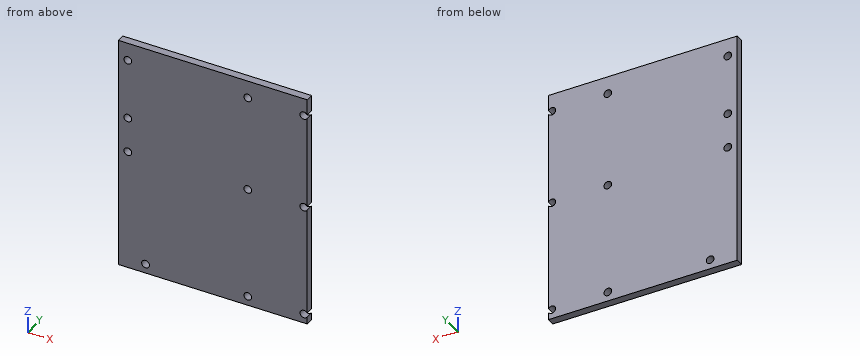
from build123d import *

# Parameters (mm, degrees)
SKETCH2_W           = 243.84
SKETCH2_H           = 304.8
BOSS_EXTRUDE1_DEPTH = 10
SKETCH1_R           = 5
CUT_EXTRUDE2_DEPTH  = 10


with BuildPart() as part:
    # Sketch2 → Boss-Extrude1 (new body)
    with BuildSketch(Plane(origin=(0, 0, 0), x_dir=(1, 0, 0), z_dir=(0, 1, 0))):
        Rectangle(SKETCH2_W, SKETCH2_H)
    extrude(amount=BOSS_EXTRUDE1_DEPTH)

    # Sketch1 → Cut-Extrude2 (cut)
    with BuildSketch(Plane(origin=(0, 0, 0), x_dir=(1, 0, 0), z_dir=(0, 1, 0))):
        with Locations((-86.9, 140.24)):
            Circle(SKETCH1_R)
        with Locations((45.18, 140.24)):
            Circle(SKETCH1_R)
        with Locations((117.57, 140.24)):
            Circle(SKETCH1_R)
        with Locations((117.57, -5.08)):
            Circle(SKETCH1_R)
        with Locations((45.18, -5.08)):
            Circle(SKETCH1_R)
        with Locations((-109.76, -5.08)):
            Circle(SKETCH1_R)
        with Locations((-109.76, -50.8)):
            Circle(SKETCH1_R)
        with Locations((-109.76, -129.196094703)):
            Circle(SKETCH1_R)
        with Locations((45.18, -129.54)):
            Circle(SKETCH1_R)
        with Locations((117.57, -129.54)):
            Circle(SKETCH1_R)
    extrude(amount=CUT_EXTRUDE2_DEPTH, mode=Mode.SUBTRACT)


solid = part.part
The model under review builds one solid part; all positions refer to its coordinate system, in mm. Round coordinates to 2 decimals unless told otherwise and drop trailing zeros. Loops run counter-clockwise (first coordinate to the right, second up) from the corner with the lowest first, then second, coordinate; pieces in that order, holes last. Notation, with made-up numbers: M -11,67 L 17,67 A16 cw 17,85 Z; hole C 9.5,27 d4. An arc over 180 degrees is marked long. Answer as a JSON object with one key per item and string values.
Item 1: For line 1 along Z through (x, y) = (117.57, 4.75); line 2 along X through (y, z) = (2, 5.08); line 3 along Z through (x, y) = (-109.76, 5.5), list the stretches that pass through material, from the lowest coordinate up.
Check sheet entries:
{"line 1": "-152.4 to -145.24, -135.24 to 0.08, 10.08 to 124.54, 134.54 to 152.4", "line 2": "-121.92 to -114.76, -104.76 to 40.18, 50.18 to 112.57", "line 3": "-152.4 to 0.08, 10.08 to 45.8, 55.8 to 124.2, 134.2 to 152.4"}
Item 2: We need section C-C, the plane x = -86.9. State the section outline as (y, z) points, and give its area (3 significant figures).
Check sheet entries:
{"outline": "M 0,-152.4 L 10,-152.4 L 10,-145.24 L 0,-145.24 Z; M 0,-135.24 L 10,-135.24 L 10,152.4 L 0,152.4 Z", "area": "2,950 mm2"}
Item 3: We need section B-B, the plane z = 50.8. State the section outline as (x, y) points.
Check sheet entries:
{"outline": "M -121.92,0 L -114.76,0 L -114.76,10 L -121.92,10 Z; M -104.76,0 L 121.92,0 L 121.92,10 L -104.76,10 Z"}
Item 4: We need section A-A, the plane x = 45.18. State the section outline as (y, z) points, and give its area (3 significant figures).
Check sheet entries:
{"outline": "M 0,-152.4 L 10,-152.4 L 10,-145.24 L 0,-145.24 Z; M 0,-135.24 L 10,-135.24 L 10,0.08 L 0,0.08 Z; M 0,10.08 L 10,10.08 L 10,124.54 L 0,124.54 Z; M 0,134.54 L 10,134.54 L 10,152.4 L 0,152.4 Z", "area": "2,750 mm2"}
